```python
from build123d import *

# Parameters (mm, degrees)
F0_W     = 105
F0_H     = 52.5
F1_DEPTH = 15
F3_DEPTH = 105.001
F6_DEPTH = 15.001
F8_DEPTH = 15.001
F9_ANGLE = 10.691248


with BuildPart() as f1:
    # F0 (on Top) → F1 (new body)
    with BuildSketch(Plane.XY):
        Rectangle(F0_W, F0_H)
    extrude(amount=F1_DEPTH)

    # F2 (on face) → F3 (cut, through all)
    with BuildSketch(Plane.YZ.offset(52.5)):
        Polygon((-26.25, 15), (-26.25, 5.088328), (26.25, 15), align=None)
        Polygon((26.25, 9.911672), (-26.25, 0), (26.25, 0), align=None)
    extrude(amount=-F3_DEPTH, mode=Mode.SUBTRACT)

    # F5 (on Top) → F6 (cut, through all)
    with BuildSketch(Plane.XY):
        Polygon((-52.5, 26.25), (-52.5, -26.25), (0, 26.25), align=None)
        Polygon((0, 26.25), (52.5, -26.25), (52.5, 26.25), align=None)
    extrude(amount=F6_DEPTH, mode=Mode.SUBTRACT)

    # F7 (on Top) → F8 (cut, through all)
    with BuildSketch(Plane.XY):
        Polygon((5, 21.25), (0, 26.25), (-5, 21.25), align=None)
    extrude(amount=F8_DEPTH, mode=Mode.SUBTRACT)


with BuildPart() as f1_1:
    # F9: moved
    add(f1.part.rotate(Axis((0, -26.25, 0), (-1, 0, 0)), F9_ANGLE))


solid = f1_1.part
```
Work out the finished part from the listing and answer in its coordinate system (mm). Coordinates: 2 decimals unless noted, no trailing zeros. Write each loop counter-clockwise with the first axis right and the second up, starting at its lowest first coordinate (ties: lowest second). Pieces come first, ordered by that corner, then holes. Notation, with made-up numbers: (83, 66.5) - (96, 66.5) arc R16 cw to (96, 91.5) - close; hole circle Ø4 at (83, 86.5). An arc over 180 degrees is marked (long way). Answer as a JSON object with one key per item and string values.
Q1. Given pin 1 Ø3 at (y, z) = (-11.5, 2) entering from -X, flat-ended and moving along its own axis, determine where the tip first touches the part or whether it passes through.
Results list:
{"pin 1": "stops at x = -39.88"}
Q2. Find section B-B (y = 15). Write down the section's boundary in (x, z), plus the area to 3 significant figures.
Results list:
{"outline": "(-12.89, 5) - (-11.97, 0) - (11.97, 0) - (12.89, 5) - close", "area": "124 mm^2"}
Q3. Find section A-A (x = -2). Write down the section's boundary in (y, z).
Results list:
{"outline": "(-26.25, 0) - (22.09, 0) - (23.03, 5) - (-25.31, 5) - close"}
Q4. Consider L1, parallel to Y at x = 15, z = 1.6; L2, parallel to Y at x = -26.5, z = 3.55; L3, parallel to X at y = -6, z = 2.2. Determine where each line is inside the solid, lowest interval first. Write a range as from..to.
Results list:
{"L1": "y = -25.95..12.21", "L2": "y = -25.58..0.88", "L3": "x = -33.01..33.01"}
